from build123d import *

# Parameters (mm, degrees)
SKETCH_1_W      = 44.92820323
SKETCH_1_H      = 44.928203231
EXTRUDE_1_DEPTH = 4
EXTRUDE_2_DEPTH = 6
EXTRUDE_3_DEPTH = 10
EXTRUDE_4_DEPTH = 9


with BuildPart() as part:
    # Эскиз1 → Бобышка-Вытянуть1 (new body)
    with BuildSketch(Plane(origin=(0, 102.195974268, 0), x_dir=(1, 0, 0), z_dir=(0, 1, 0))):
        Polygon((6.758980694, -68.473129836), (1.558980694, -68.473129836), (1.558980694, -110.573129836), (6.758980694, -110.573129836), (11.758980694, -122.773129836), (11.758980694, -130.773129836), (117.858980694, -130.773129836), (117.858980694, -122.773129836), (122.858980694, -110.573129836), (128.058980694, -110.573129836), (128.058980694, -68.473129836), (122.858980694, -68.473129836), (117.858980694, -56.273129836), (117.858980694, -48.273129836), (11.758980694, -48.273129836), (11.758980694, -56.273129836), align=None)
        with Locations((64.808980694, -89.523129837)):
            Rectangle(SKETCH_1_W, SKETCH_1_H, mode=Mode.SUBTRACT)
    extrude(amount=EXTRUDE_1_DEPTH)

    # Эскиз2 → Бобышка-Вытянуть2 (add)
    with BuildSketch(Plane(origin=(0, 106.195974268, 0), x_dir=(1, 0, 0), z_dir=(0, 1, 0))):
        with BuildLine():
            Line((95.642201414, -130.773129836), (117.858980694, -130.773129836))
            Line((117.858980694, -130.773129836), (117.858980694, -122.773129836))
            Line((117.858980694, -122.773129836), (122.858980694, -110.573129836))
            Line((122.858980694, -110.573129836), (128.058980694, -110.573129836))
            Line((128.058980694, -110.573129836), (128.058980694, -68.473129836))
            Line((128.058980694, -68.473129836), (122.858980694, -68.473129836))
            Line((122.858980694, -68.473129836), (117.858980694, -56.273129836))
            Line((117.858980694, -56.273129836), (117.858980694, -48.273129836))
            Line((117.858980694, -48.273129836), (95.642201414, -48.273129836))
            ThreePointArc((95.642201414, -48.273129836), (116.308980694, -89.523129836), (95.642201414, -130.773129836))
        make_face()
        with BuildLine():
            Line((33.975759973, -48.273129836), (11.758980694, -48.273129836))
            Line((11.758980694, -48.273129836), (11.758980694, -56.273129836))
            Line((11.758980694, -56.273129836), (6.758980694, -68.473129836))
            Line((6.758980694, -68.473129836), (1.558980694, -68.473129836))
            Line((1.558980694, -68.473129836), (1.558980694, -110.573129836))
            Line((1.558980694, -110.573129836), (6.758980694, -110.573129836))
            Line((6.758980694, -110.573129836), (11.758980694, -122.773129836))
            Line((11.758980694, -122.773129836), (11.758980694, -130.773129836))
            Line((11.758980694, -130.773129836), (33.975759973, -130.773129836))
            ThreePointArc((33.975759973, -130.773129836), (13.308980694, -89.523129836), (33.975759973, -48.273129836))
        make_face()
    extrude(amount=EXTRUDE_2_DEPTH)

    # Эскиз3 → Бобышка-Вытянуть3 (add)
    with BuildSketch(Plane(origin=(0, 112.195974268, 0), x_dir=(1, 0, 0), z_dir=(0, 1, 0))):
        with BuildLine():
            Line((1.558980694, -130.773129836), (1.558980694, -48.273129836))
            Line((1.558980694, -48.273129836), (33.975759973, -48.273129836))
            ThreePointArc((33.975759973, -48.273129836), (13.308980694, -89.523129836), (33.975759973, -130.773129836))
            Line((33.975759973, -130.773129836), (1.558980694, -130.773129836))
        make_face()
        with BuildLine():
            Line((95.642201414, -48.273129836), (128.058980694, -48.273129836))
            Line((128.058980694, -48.273129836), (128.058980694, -130.773129836))
            Line((128.058980694, -130.773129836), (95.642201414, -130.773129836))
            ThreePointArc((95.642201414, -130.773129836), (116.308980694, -89.523129836), (95.642201414, -48.273129836))
        make_face()
    extrude(amount=EXTRUDE_3_DEPTH)

    # Эскиз4 → Бобышка-Вытянуть4 (add)
    with BuildSketch(Plane(origin=(0, 122.195974268, 0), x_dir=(1, 0, 0), z_dir=(0, 1, 0))):
        Polygon((1.558980694, -48.273129836), (16.558980694, -48.273129836), (16.558980694, -54.273129836), (7.558980694, -63.273129836), (1.558980694, -63.273129836), align=None)
        Polygon((128.058980694, -48.273129836), (113.058980694, -48.273129836), (113.058980694, -54.273129836), (122.058980694, -63.273129836), (128.058980694, -63.273129836), align=None)
        Polygon((128.058980694, -130.773129836), (128.058980694, -115.773129836), (122.058980694, -115.773129836), (113.058980694, -124.773129836), (113.058980694, -130.773129836), align=None)
        Polygon((1.558980694, -130.773129836), (1.558980694, -115.773129836), (7.558980694, -115.773129836), (16.558980694, -124.773129836), (16.558980694, -130.773129836), align=None)
    extrude(amount=EXTRUDE_4_DEPTH)


solid = part.part
Read the model definition and answer for the solid it produces. Units are mm, in the model's axes. A direction names the side the tool comes from. Give positions to 0.01 mm unless a question says otherwise; leave off trailing zeros. Write each loop counter-clockwise with the first axis right and the second up, starting at its lowest first coordinate (ties: lowest second). Pieces come first, ordered by that corner, then holes. Notation, with made-up numbers: (-26, 69.25) - (19, 69.25) arc R27 cw to (19, 99.25) - close; hole circle Ø5 at (-28.5, -4). An arc over 180 degrees is marked (long way). Use CSV: the item, a comma, the result in double quotes. Start each with the question number.
(1) Determine the mould class of faces 1 (the flat face through (117.859, 107, 127)), 2 (the flat face through (5, 127, 63.273)), 3 (the flat face through (119, 122.196, 89)) for opening direction X: +X half, -X half, draft (parallel to the pull), parting line (faces both ways), or undercut.
(2) Consider line 1 along Z through (x, y) = (7, 125); line 2 along Y through (x, z) = (79, 116); line 3 along Y through (x, z) = (122.5, 118.5). Determine where each line is inside the solid, lowest interval first.
(3) Given P1, Ø5.5, axis at x = 5, y = 108.5, coming from the +Z side; P2, Ø2.5, axis at y = 108, z = 51, coming from the +X side; P3, Ø4, axis at y = 109.5, z = 126.5, coming from the -X side, each flat-ended and moving along its own axis, determine where each tip first touches the part or whether it passes through.
(4) For faces 4 (the flat face through (87.273, 104, 90)), 5 (the flat face through (9.294, 107.126, 62.288)), 6 (the flat face through (5, 127, 115.773)), 7 (the flat face through (6, 112.196, 121)), 8 (the flat face through (117.859, 107, 52)), determine the directions among +Z, -Z, +X, -X, +Y, -Y from which every point of the face is accessible in a straight line to the end or side of a thin tool.
(5) Find section C-C (y = 108). Give the vertices of the cut face in (x, z), plus the area to 3 significant figures.
(6) Find section A-A (y = 126). Give the vertices of the cut face in (x, z), plus the area to 3 significant figures.
(7) Find section B-B (x = 53). Give the vertices of the cut face in (y, z).
(8) Find section D-D (z = 101). Give the vertices of the cut face in (x, y), plus the area to 3 significant figures.
Findings below:
1,face 1,"+X half"
1,face 2,"draft"
1,face 3,"undercut"
2,line 1,"48.27 to 63.27, 115.77 to 130.77"
2,line 2,"102.2 to 106.2"
2,line 3,"112.2 to 131.2"
3,P1,"z = 112.99"
3,P2,"x = 117.86"
3,P3,"x = 11.76"
4,face 4,"+Y, -Y"
4,face 5,"-Z, -X, -Y"
4,face 6,"+X, -X, +Y"
4,face 7,"+Z, -X, -Y"
4,face 8,"-Z, +X, -Y"
5,outline,"(1.56, 68.47) - (6.76, 68.47) - (11.76, 56.27) - (11.76, 48.27) - (33.98, 48.27) arc R51.5 cw to (33.98, 130.77) - (11.76, 130.77) - (11.76, 122.77) - (6.76, 110.57) - (1.56, 110.57) - close; (95.64, 48.27) - (117.86, 48.27) - (117.86, 56.27) - (122.86, 68.47) - (128.06, 68.47) - (128.06, 110.57) - (122.86, 110.57) - (117.86, 122.77) - (117.86, 130.77) - (95.64, 130.77) arc R51.5 cw to start"
5,area,"2,260 mm2"
6,outline,"(1.56, 48.27) - (16.56, 48.27) - (16.56, 54.27) - (7.56, 63.27) - (1.56, 63.27) - close; (1.56, 115.77) - (7.56, 115.77) - (16.56, 124.77) - (16.56, 130.77) - (1.56, 130.77) - close; (113.06, 48.27) - (128.06, 48.27) - (128.06, 63.27) - (122.06, 63.27) - (113.06, 54.27) - close; (113.06, 124.77) - (122.06, 115.77) - (128.06, 115.77) - (128.06, 130.77) - (113.06, 130.77) - close"
6,area,"738 mm2"
7,outline,"(102.2, 48.27) - (106.2, 48.27) - (106.2, 67.06) - (102.2, 67.06) - close; (102.2, 111.99) - (106.2, 111.99) - (106.2, 130.77) - (102.2, 130.77) - close"
8,outline,"(1.56, 102.2) - (42.34, 102.2) - (42.34, 106.2) - (14.6, 106.2) - (14.6, 122.2) - (1.56, 122.2) - close; (87.27, 102.2) - (128.06, 102.2) - (128.06, 122.2) - (115.01, 122.2) - (115.01, 106.2) - (87.27, 106.2) - close"
8,area,"744 mm2"
